Autodesk Inventor part; units mm, degrees
ref_plane "Work Plane4" through (0, 0, 20) normal (0, 0, -1) x (1, 0, 0)
ref_plane "YZ Plane" through (0, 0, 0) normal (1, 0, 0) x (0, 1, 0)
ref_plane "XZ Plane" through (0, 0, 0) normal (0, 1, 0) x (-1, 0, 0)
sketch "Sketch1" plane through (0, 0, 0) normal (1, 0, 0) x (0, 1, 0)
  line L0 (-20, 20) -> (20, 20)
  line L1 (20, 20) -> (20, -20)
  line L2 (20, -20) -> (-20, -20)
  line L3 (-20, -20) -> (-20, 20)
  line L4 (-20, 20) -> (20, -20) construction
  line L5 (20, 20) -> (-20, -20) construction
  point P0 (0, 0)
  dimension "d0" = 40
  dimension "d1" = 40
extrude "Extrusion1" add sketch "Sketch1" along normal mid plane 6
sketch "Sketch2" plane through (3, 0, 0) normal (1, 0, 0) x (0, 0, -1)
  line L0 (20, 20) -> (-20, 20)
  line L1 (-20, 20) -> (-15, 20)
  line L2 (-15, 20) -> (-15, 15)
  line L3 (-15, 15) -> (-20, 15)
  line L4 (-20, 20) -> (-20, -20)
  circle A0 centre (-15, 15) radius 3
  point P0 (0, 0)
  dimension "d4" = 5
  dimension "d5" = 5
  dimension "d6" = 6
extrude "Extrusion2" cut sketch "Sketch2" against normal blind 6 contours A0 L3 L2 | L2 L3 A0
mirror "Mirror1" about plane through (0, 0, 0) normal (0, 0, 1) of "Extrusion2"
mirror "Mirror2" about plane through (0, 0, 0) normal (0, 1, 0) of "Extrusion2", "Mirror1"
ref_plane "Work Plane4" through (0, 0, 20) normal (0, 0, -1) x (1, 0, 0)
ref_plane "Work Plane3" through (0, 0, 0) normal (0, 0, -1) x (1, 0, 0)
sketch "Sketch3" plane through (0, 0, 20) normal (0, 0, -1) x (1, 0, 0)
  line L0 (3, -20) -> (3, 20)
  line L1 (3, 0) -> (3, -15)
  line L2 (3, -15) -> (153, -15) construction
  line L3 (3, 0) -> (3, -7.5)
  point P0 (0, 0)
  dimension "d10" = 15
  dimension "bracketlength" = 150
  dimension "d12" = 7.5
sketch "Sketch4" plane through (3, 0, 0) normal (1, 0, 0) x (0, 0, -1)
  circle A0 centre (-15, 15) radius 3
  circle A1 centre (15, 15) radius 3
  circle A2 centre (-15, 15) radius 3
  circle A3 centre (-15, 15) radius 3
  circle A4 centre (15, 15) radius 3
  line L0 (-20, 20) -> (20, 20)
  line L1 (-16.0857, 20) -> (-12.9984, 17.2346)
  line L2 (-17.7822, 15) -> (18, 15)
  circle A5 centre (15, 15) radius 3
  line L3 (-16.0857, 10) -> (-12.9984, 12.7654)
  line L4 (0, 20) -> (0, 0)
  line L5 (-16.0857, 10) -> (-20, 6.4938)
  line L6 (-20, -20) -> (-20, 20)
  line L7 (-20, 6.4938) -> (-20, 0)
  circle A6 centre (15, 15) radius 3
  line L8 (16.0857, 20) -> (12.9984, 17.2346)
  line L9 (16.0857, 10) -> (12.9984, 12.7654)
  line L10 (16.0857, 10) -> (20, 6.4938)
  line L11 (20, 6.4938) -> (20, 0)
  line L12 (-16.0857, 20) -> (16.0857, 20)
  line L13 (-20, 0) -> (20, 0)
extrude "Extrusion3" add sketch "Sketch4" along normal blind 150 contours L2 L4 L13 L6 L5 L3 A0 | A0 L1 L0 L4 L2 | L4 L0 L8 A1 L2 | L2 A1 L9 L10 L11 L13 L4
sketch "Sketch5" plane through (3, 0, -20) normal (0, -1, 0) x (1, 0, 0)
  line L0 (150, 0) -> (150, 40)
  line L1 (150, 40) -> (150, 50)
  line L2 (150, 50) -> (150, -10)
  line L3 (150, 3.9143) -> (150, 36.0857)
  line L4 (150, 20) -> (110, 20)
  circle A0 centre (130, 20) radius 50
  point P0 (-3, 20)
  dimension "d15" = 10
  dimension "d16" = 60
  dimension "d17" = 40
  dimension "panmotorholderdiam" = 100
extrude "Extrusion4" add sketch "Sketch5" along normal blind 80
sketch "Sketch6" plane through (133, -80, 0) normal (0, -1, 0) x (1, 0, 0)
  circle A0 centre (0, 0) radius 46.5
  point P0 (-133, 0)
  dimension "d21" = 93
extrude "Extrusion5" cut sketch "Sketch6" against normal blind 70
ref_plane "Work Plane1" through (0, 0, 0) normal (0, 0, 1) x (1, 0, 0)
ref_plane "Work Plane2" through (0, 0, 0) normal (0, 0, -1) x (1, 0, 0)
properties part number "TopBracket" material "ABS Plastic"
Could you check a few things on this model? Use its own coordinates, in mm. A direction names the side the tool comes from. Coordinates: 2 decimals unless noted, no trailing zeros. Order: outer loops, then holes, each group sorted by start corner. A loop starts at its lowest first (then second) coordinate and runs counter-clockwise, first axis right, second up. Notation, with made-up numbers: (11, -22) -> (31, -22) arc R11 cw to (31, -5) -> close; hole circle Ø2 at (28, 69.25). An arc over 180 degrees is marked (long way). One line per item, written item: value. Start each with the question number.
1) Which directions (+Z, -Z, +X, -X, +Y, -Y) give clear straight access to the entire face, cutting with the end or side of a thin tool? Please do faces 1 (the flat face through (153, 10, 0)), 2 (the cylindrical face through (0, -16.8, 17.4)), 3 (the flat face through (0, -20, 0)), 4 (the flat face through (3, -10, 0)), 5 (the cylindrical face through (86.545, -45.49, 2.045)).
2) Imagine slicing it at C-C on x = 52. List the corners of the cut face in (y, z) for me, plus the area to 3 significant figures.
3) I'm going to push flat-ended pins straight in: pin 1 (2 mm diameter, centred on y = -6.5, z = 26, fed in from +X); pin 2 (9.5 mm diameter, centred on y = -15, z = -15, fed in from +X); pin 3 (7.5 mm diameter, centred on y = 15, z = -15.5, fed in from +X); pin 4 (7 mm diameter, centred on y = -15, z = 15, fed in from -X). Where does each tip first touch, or does it pass through?
4) Imagine slicing it at B-B on z = 0. List the corners of the cut face in (x, y) for me.
5) If I drill on L1, parallel to Z at x = 1.6, y = -15; L2, parallel to X at y = -7, z = 2, over which ranges is the centre line in solid material (lowest first)? Write a range as [from, to].
6) We'd pull the mould along X, two halves only. Please class faces 6 (the flat face through (74, 20, 0)), 7 (the flat face through (44, 0, 0)), 8 (the flat face through (3, 13, -18)), 9 (the flat face through (-3, 0, 0)): +X half, -X half, draft (parallel to the pull), parting line (faces both ways), or undercut.
7) Imagine slicing it at D-D on y = -40. List the corners of the cut face in (x, z) for me, plus the area to 3 significant figures.
8) Imagine slicing it at A-A on y = -15. List the corners of the cut face in (x, z) for me, plus the area to 3 significant figures.
Answer list:
1. face 1: +Z, -Z, +X, +Y
1. face 2: -X
1. face 3: +Z, -Z, -X, -Y
1. face 4: +Z, -Z, -Y
1. face 5: -Y
2. outline: (0, -20) -> (6.49, -20) -> (10, -16.09) -> (12.77, -13) arc R3 cw to (17.23, -13) -> (20, -16.09) -> (20, 16.09) -> (17.23, 13) arc R3 cw to (12.77, 13) -> (10, 16.09) -> (6.49, 20) -> (0, 20) -> close
2. area: 657 mm2
3. pin 1: stops at x = 176.3
3. pin 2: stops at x = 181.94
3. pin 3: stops at x = 153
3. pin 4: stops at x = -3
4. outline: (-3, -20) -> (3, -20) -> (3, 0) -> (83, 0) -> (83, -80) -> (86.5, -80) -> (86.5, -10) -> (179.5, -10) -> (179.5, -80) -> (183, -80) -> (183, 0) -> (153, 0) -> (153, 20) -> (-3, 20) -> close
5. L1: z = [-20, -18], [-12, 12], [18, 20]
5. L2: x = [-3, 3], [83.04, 182.96]
6. face 6: draft
6. face 7: undercut
6. face 8: +X half
6. face 9: -X half
7. outline: circle Ø100 at (133, 0); hole circle Ø93 at (133, 0)
7. area: 1,060 mm2
8. outline: (-3, -20) -> (3, -20) -> (3, -18) -> (-3, -18) -> close; (-3, -12) -> (3, -12) -> (3, 12) -> (-3, 12) -> close; (-3, 18) -> (3, 18) -> (3, 20) -> (-3, 20) -> close; circle Ø100 at (133, 0); hole circle Ø93 at (133, 0)
8. area: 1,230 mm2
